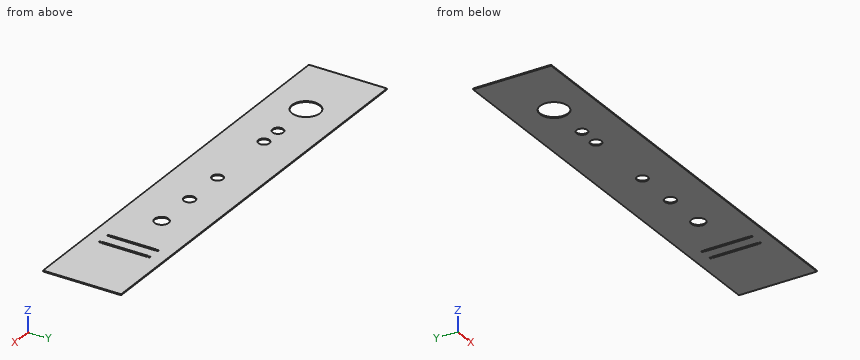
Autodesk Inventor part; units mm, degrees
ref_plane "YZ Plane" through (0, 0, 0) normal (1, 0, 0) x (0, 1, 0)
ref_plane "XZ Plane" through (0, 0, 0) normal (0, 1, 0) x (-1, 0, 0)
ref_plane "XY Plane" through (0, 0, 0) normal (0, 0, 1) x (1, 0, 0)
sketch "Sketch1" plane through (0, 0, 0) normal (0, 0, 1) x (1, 0, 0)
  line L0 (-241.3, -44.45) -> (241.3, -44.45)
  line L1 (241.3, -44.45) -> (241.3, 44.45)
  line L2 (241.3, 44.45) -> (-241.3, 44.45)
  line L3 (-241.3, 44.45) -> (-241.3, -44.45)
  point P0 (0, 0)
  dimension "d0" = 482.6
  dimension "d1" = 88.9
  dimension "d62" = 44.45
  dimension "d63" = 241.3
extrude "Extrusion1" add sketch "Sketch1" along normal blind 1.1113
sketch "Sketch3" plane through (0, 0, 1.1113) normal (0, 0, 1) x (1, 0, 0)
  point P0 (0, 0)
sketch "Sketch4" plane through (0, 0, 1.1113) normal (0, 0, 1) x (1, 0, 0)
  line L0 (147.7124, 26.0031) -> (150.1, 26.0031)
  line L1 (150.1, 26.0031) -> (150.1, -25.9969)
  line L2 (150.1, -25.9969) -> (147.7124, -25.9969)
  line L3 (147.7124, -25.9969) -> (147.7124, 26.0031)
  line L4 (162.7124, 26.0031) -> (165.1, 26.0031)
  line L5 (165.1, 26.0031) -> (165.1, -25.9969)
  line L6 (165.1, -25.9969) -> (162.7124, -25.9969)
  line L7 (162.7124, -25.9969) -> (162.7124, 26.0031)
  line L8 (-241.3, -44.45) -> (241.3, -44.45)
  line L9 (241.3, -44.45) -> (241.3, 44.45)
  circle A0 centre (-114.3, 0) radius 6.2484
  circle A1 centre (-88.9, 0) radius 6.2484
  circle A2 centre (-4.6876, 0) radius 6.2484
  circle A3 centre (46.1124, 0) radius 6.5
  circle A4 centre (96.9124, 0) radius 8
  line L10 (241.3, 44.45) -> (-241.3, 44.45)
  line L11 (-241.3, -44.45) -> (241.3, -44.45)
  line L12 (241.3, -44.45) -> (241.3, 44.45)
  line L13 (241.3, 44.45) -> (-241.3, 44.45)
  line L14 (-241.3, 44.45) -> (-241.3, -44.45)
  circle A5 centre (163.9062, 28.0031) radius 1.05
  circle A6 centre (163.9062, -27.9969) radius 1.05
  circle A7 centre (148.9062, 28.0031) radius 1.05
  circle A8 centre (148.9062, -27.9969) radius 1.05
  circle A9 centre (-165.1, 0) radius 15.875
  line L15 (148.9062, 26.0031) -> (148.9062, -25.9969)
  line L16 (163.9062, 26.0031) -> (163.9062, -25.9969)
  point P0 (0, 0)
  dimension "d9" = 2.3876
  dimension "d12" = 2.3876
  dimension "d13" = 52
  dimension "d17" = 18.4531
  dimension "d18" = 52
  dimension "d20" = 18.4531
  dimension "d22" = 12.4968
  dimension "d23" = 12.4968
  dimension "d24" = 12.4968
  dimension "d26" = 13
  dimension "d27" = 16
  dimension "d28" = 50.8
  dimension "d35" = 44.45
  dimension "d36" = 44.45
  dimension "d38" = 44.45
  dimension "d40" = 44.45
  dimension "d42" = 50.8
  dimension "d47" = 2.1
  dimension "d48" = 2.1
  dimension "d49" = 56
  dimension "d50" = 2
  dimension "d53" = 2.1
  dimension "d54" = 2.1
  dimension "d55" = 56
  dimension "d58" = 2
  dimension "d59" = 76.2
  dimension "d65" = 31.75
  dimension "d66" = 25.4
  dimension "d67" = 44.45
  dimension "d68" = 50.8
  dimension "d69" = 76.2
  dimension "d70" = 44.45
  dimension "d71" = 50.8
  dimension "d74" = 15
  dimension "d75" = 0
  dimension "d76" = 0
  dimension "d77" = 0
  dimension "d78" = 0
extrude "Extrusion3" cut sketch "Sketch4" against normal up to next contours L0 L15 L2 L3 | L0 L1 L2 L15 | L4 L16 L6 L7 | L4 L5 L6 L16 | A0 | A1 | A2 | A3 | A4 | A5 | A6 | A7 | A8 | A9
properties part number "Faceplate"
Could you check a few things on this model? Use its own coordinates, in mm. Give positions to 0.01 mm unless a question says otherwise; leave off trailing zeros. Order: outer loops, then holes, each group sorted by start corner. A loop starts at its lowest first (then second) coordinate and runs counter-clockwise, first axis right, second up. Notation, with made-up numbers: (48, 11) -> (102, 11) arc R17 ccw to (102, 31) -> close; hole circle Ø2 at (18.25, -22). An arc over 180 degrees is marked (long way). Return JSON: item names as keys, results as strings.
1. Imagine slicing it at B-B on x = -165.1. List the corners of the cut face in (y, z) for me (3 decimals).
Answer list:
{"outline": "(-44.45, 0) -> (-15.875, 0) -> (-15.875, 1.111) -> (-44.45, 1.111) -> close; (15.875, 0) -> (44.45, 0) -> (44.45, 1.111) -> (15.875, 1.111) -> close"}
2. I need wall thicknesses on line 1 (X direction, y = 24.5, z = 0.1); line 2 (Y direction, x = 149, z = 0.9); line 3 (Y direction, x = -179, z = 0.85). Which ranges of each line are inside material? Lowest first, please. Write a range as from..to.
Answer list:
{"line 1": "x = -241.3..147.71, 150.1..162.71, 165.1..241.3", "line 2": "y = -44.45..-29.04, -26.95..-26, 26..26.96, 29.05..44.45", "line 3": "y = -44.45..-7.67, 7.67..44.45"}
3. Imagine slicing it at A-A on x = -114.3. List the corners of the cut face in (y, z) for me.
Answer list:
{"outline": "(-44.45, 0) -> (-6.25, 0) -> (-6.25, 1.11) -> (-44.45, 1.11) -> close; (6.25, 0) -> (44.45, 0) -> (44.45, 1.11) -> (6.25, 1.11) -> close"}
4. Imagine slicing it at C-C on y = 0. Give the number of separate pieces and of enclosed holes in the cut face, then the cut area to 3 significant figures.
Answer list:
{"separate pieces": "9", "enclosed holes": "0", "area": "422 mm2"}
